Could you check a few things on this drawing? It's one solid part, dimensions in mm from its lowest x, y, z. Round coordinates to 2 decimals unless told otherwise and drop trailing zeros. Order: outer loops, then holes, each group sorted by start corner. A loop starts at its lowest first (then second) coordinate and runs counter-clockwise, first axis right, second up. Notation, with made-up numbers: (7.5, 31.5) -> (54.5, 31.5) arc R15 ccw to (54.5, 53.5) -> close; hole circle Ø5 at (48, 82.5). An arc over 180 degrees is marked (long way). Use a Markdown table: item, result. Add a question column.
(1) I want a section at D-D, the plane y = 2.5. Please give me the cut outline in (x, z).
(2) I'm going to push flat-ended pins straight in: P1, Ø16, axis at x = 97.5, z = 97.5, coming from the -Y side; P2, Ø10, axis at x = 143, y = 21.5, coming from the -Z side; P3, Ø2.5, axis at x = 55.5, z = 97, coming from the +Y side; P4, Ø1, axis at y = 8, z = 105, coming from the -X side. Where does each tip first touch, or does it pass through?
(3) If I drill on probe 1 along X at (y, z) = (18.75, 97.5) (1 decimal); probe 2 along Z at (x, y) = (100, 16); probe 3 along Z at (x, y) = (84, 14.5), over which ranges is the centre line in solid material (lowest first)?
(4) I want a section at C-C, the plane y = 21. Please give me the cut outline in (x, z) (1 decimal), then the cut area to 3 significant figures.
(5) I want a section at B-B, the plane z = 97.5. Please give me the cut outline in (x, y) (1 decimal).
(6) I want a section at A-A, the plane x = 97.5. Please give me the cut outline in (y, z), then the cut area to 3 significant figures.
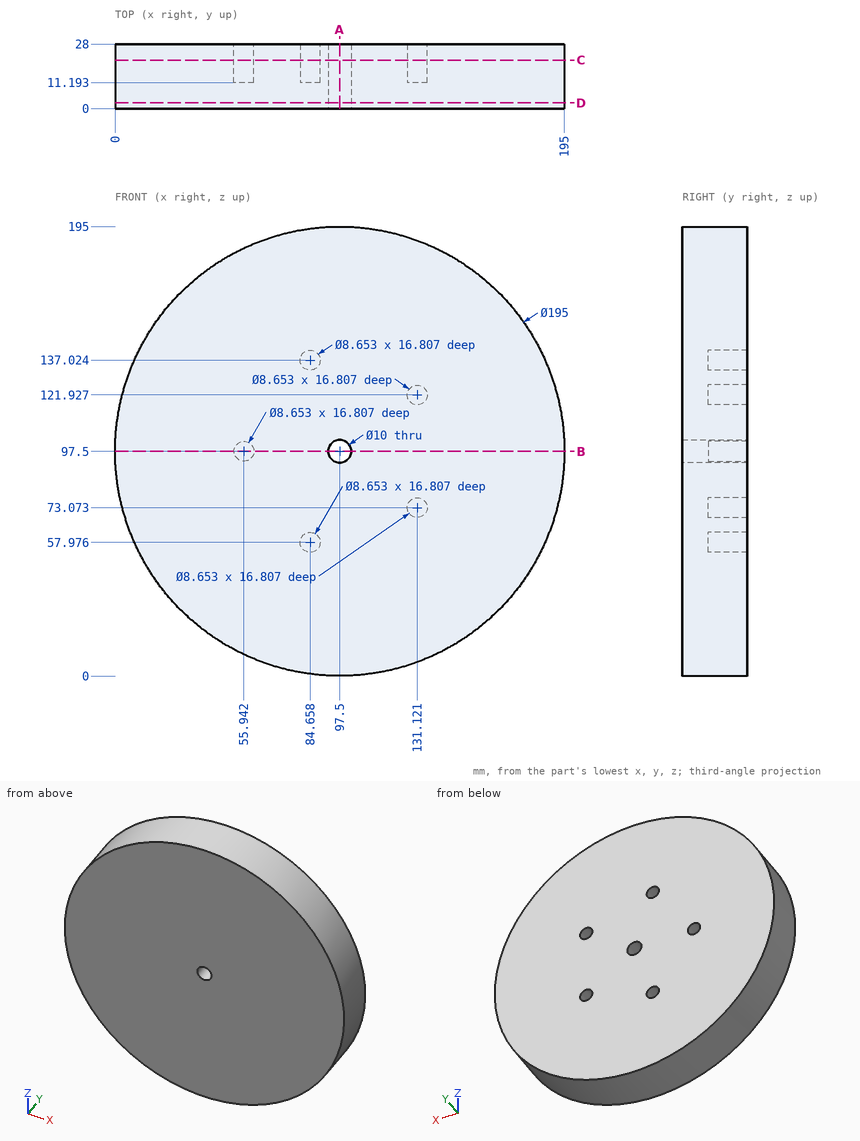
Taken from the geometry:
| question | item | result |
|---|---|---|
| 1 | outline | circle Ø195 at (97.5, 97.5); hole circle Ø10 at (97.5, 97.5) |
| 2 | P1 | stops at y = 0 |
| 2 | P2 | stops at z = 8.81 |
| 2 | P3 | stops at y = 11.19 |
| 2 | P4 | stops at x = 0.25 |
| 3 | probe 1 | x = 0 to 51.6, 60.3 to 92.5, 102.5 to 195 |
| 3 | probe 2 | z = 0.03 to 93.17, 101.83 to 194.97 |
| 3 | probe 3 | z = 0.94 to 53.7, 62.25 to 132.75, 141.3 to 194.06 |
| 4 | outline | circle Ø195 at (97.5, 97.5); hole circle Ø8.7 at (55.9, 97.5); hole circle Ø8.7 at (84.7, 58); hole circle Ø8.7 at (84.7, 137); hole circle Ø10 at (97.5, 97.5); hole circle Ø8.7 at (131.1, 73.1); hole circle Ø8.7 at (131.1, 121.9) |
| 4 | area | 29,500 mm2 |
| 5 | outline | (0, 0) -> (92.5, 0) -> (92.5, 28) -> (60.3, 28) -> (60.3, 11.2) -> (51.6, 11.2) -> (51.6, 28) -> (0, 28) -> close; (102.5, 0) -> (195, 0) -> (195, 28) -> (102.5, 28) -> close |
| 6 | outline | (0, 0) -> (28, 0) -> (28, 92.5) -> (0, 92.5) -> close; (0, 102.5) -> (28, 102.5) -> (28, 195) -> (0, 195) -> close |
| 6 | area | 5,180 mm2 |
